Could you check a few things on this model? Use its own coordinates, in mm. A direction names the side the tool comes from. Round coordinates to 2 decimals unless told otherwise and drop trailing zeros. Write each loop counter-clockwise with the first axis right and the second up, starting at its lowest first coordinate (ties: lowest second). Pieces come first, ordered by that corner, then holes.
```python
from build123d import *

# Parameters (mm, degrees)
EXTRUDE_1_DEPTH     = 25
SKETCH_2_R          = 1.75
CUT_EXTRUDE_1_DEPTH = 34
SHELL_1_T           = -2
FILLET_1_R          = 10
FILLET_2_R          = 3
FILLET_3_R          = 5
SKETCH_4_W          = 82
SKETCH_4_H          = 126.745531776
CUT_EXTRUDE_2_DEPTH = 23
FILLET_4_R          = 2
SKETCH_5_W          = 173.89587329
SKETCH_5_H          = 52
CUT_EXTRUDE_3_DEPTH = 23
FILLET_5_R          = 2
SKETCH_6_R          = 4
EXTRUDE_2_DEPTH     = 4
SKETCH_7_R          = 2.5
CUT_EXTRUDE_4_DEPTH = 6
FILLET_6_R          = 5


with BuildPart() as part:
    # Эскиз1 → Бобышка-Вытянуть1 (new body)
    with BuildSketch(Plane.XY):
        Polygon((-52.5, 30), (-45, 37.5), (45, 37.5), (52.5, 30), (52.5, -30), (45, -37.5), (-45, -37.5), (-52.5, -30), align=None)
    extrude(amount=EXTRUDE_1_DEPTH)

    # Эскиз2 → Вырез-Вытянуть1 (cut)
    with BuildSketch(Plane.XY.offset(25)):
        with Locations((-45.214466094, 30.214466094)):
            Circle(SKETCH_2_R)
        with Locations(Location((45.214466094, 30.214466094, 0), (0, 0, 180))):
            Circle(SKETCH_2_R)
        with Locations((45.214466094, -30.214466094)):
            Circle(SKETCH_2_R)
        with Locations(Location((-45.214466094, -30.214466094, 0), (0, 0, 180))):
            Circle(SKETCH_2_R)
    extrude(amount=-CUT_EXTRUDE_1_DEPTH, mode=Mode.SUBTRACT)

    # Оболочка1
    shell_1_openings = [part.faces().sort_by_distance(p)[0] for p in [
        (0, 0, 25),
    ]]
    offset(amount=SHELL_1_T, openings=shell_1_openings, kind=Kind.INTERSECTION)

    # Скругление1
    # the kernel refuses this fillet: 10 mm, written as the material it adds along each edge
    with BuildSketch(Plane(origin=(-45.74479618, -33.926776695, 2), x_dir=(0.7071067811865442, -0.7071067811865507, 0), z_dir=(0, 0, 1)), Plane(origin=(48.926776695, -30.74479618, 2), x_dir=(0.7071067811865482, 0.7071067811865467, 0), z_dir=(0, 0, 1)), Plane(origin=(45.74479618, 33.926776695, 2), x_dir=(-0.707106781186546, 0.7071067811865492, 0), z_dir=(0, 0, 1)), Plane(origin=(-48.926776695, 30.74479618, 2), x_dir=(-0.7071067811865508, -0.7071067811865444, 0), z_dir=(0, 0, 1))) as fillet_1_piece_1:
        with BuildLine():
            CenterArc((11.477032042, 3.794412555), FILLET_1_R, 183.312134334, 18.986942704)
            Line((1.493736012, 3.21665797), (1.294070091, 3.205102878))
            ThreePointArc((1.294070091, 3.205102878), (0.969771845, 1.504817982), (-0.12, 0.16))
            Line((-0.12, 0.16), (0, -0.2))
            ThreePointArc((0, -0.2), (1.112436867, -0.2), (2.039830568, -0.075888251))
            Line((2.039830568, -0.075888251), (2.224873734, 0))
        make_face()
    extrude(amount=23)
    with BuildSketch(Plane(origin=(-48.926776695, -30.74479618, 2), x_dir=(0.34351243985929386, 0.9391481265816991, 0), z_dir=(0, 0, 1)), Plane(origin=(45.74479618, -33.926776695, 2), x_dir=(-0.9391481265817004, 0.34351243985929, 0), z_dir=(0, 0, 1)), Plane(origin=(48.926776695, 30.74479618, 2), x_dir=(-0.3435124398592874, -0.9391481265817014, 0), z_dir=(0, 0, 1)), Plane(origin=(-45.74479618, 33.926776695, 2), x_dir=(0.9391481265817011, -0.34351243985928803, 0), z_dir=(0, 0, 1))) as fillet_1_piece_2:
        with BuildLine():
            CenterArc((8.275322434, 8.811292173), FILLET_1_R, 222.791938952, 18.986942704)
            Line((0.937067943, 2.017911495), (0.790302854, 1.882043882))
            ThreePointArc((0.790302854, 1.882043882), (0.287138375, 1.093191354), (-0.181395597, 0.084235607))
            Line((-0.181395597, 0.084235607), (0.094575114, -0.176225843))
            ThreePointArc((0.094575114, -0.176225843), (1.773283379, 0.245765435), (3.451991644, -0.176225843))
            Line((3.451991644, -0.176225843), (3.546566758, 0))
        make_face()
    extrude(amount=23)

    # Скругление2
    fillet_2_edges = [part.edges().sort_by_distance(p)[0] for p in [
        (-50.5, 29.171572875, 13.5),
        (-44.171572875, 35.5, 13.5),
        (-44.171572875, -35.5, 13.5),
        (-50.5, -29.171572875, 13.5),
        (44.171572875, -35.5, 13.5),
        (50.5, -29.171572875, 13.5),
        (50.5, 29.171572875, 13.5),
        (44.171572875, 35.5, 13.5),
    ]]
    fillet(fillet_2_edges, radius=FILLET_2_R)

    # Скругление3
    fillet_3_edges = [part.edges().sort_by_distance(p)[0] for p in [
        (45, 37.5, 12.5),
        (52.5, 30, 12.5),
        (52.5, -30, 12.5),
        (45, -37.5, 12.5),
        (-45, -37.5, 12.5),
        (-52.5, -30, 12.5),
        (-52.5, 30, 12.5),
        (-45, 37.5, 12.5),
    ]]
    fillet(fillet_3_edges, radius=FILLET_3_R)

    # Эскиз4 → Вырез-Вытянуть2 (cut)
    with BuildSketch(Plane.XY.offset(25)):
        Rectangle(SKETCH_4_W, SKETCH_4_H)
    extrude(amount=-CUT_EXTRUDE_2_DEPTH, mode=Mode.SUBTRACT)

    # Скругление4
    # the kernel refuses this fillet: 2 mm, written as the material it takes off along each edge
    with BuildSketch(Plane(origin=(41, -34.605706623, 2), x_dir=(0, -1, 0), z_dir=(0, 0, 1)), Plane(origin=(41, 34.605706623, 26.756559814), x_dir=(0, 1, 0), z_dir=(0, 0, -1))) as fillet_4_piece_1:
        with BuildLine():
            CenterArc((0.702623926, 2), FILLET_4_R, 235.828901177, 34.171098823)
            ThreePointArc((-0.420708294, 0.345272009), (-0.20250821, 0.18219615), (0, 0))
            Line((0, 0), (0.702623926, 0))
        make_face()
    extrude(amount=24.756559814, mode=Mode.SUBTRACT)
    with BuildSketch(Plane(origin=(41, -37.5, 30.118447555), x_dir=(0.9999997651545144, 0.0006853400003404547, 0), z_dir=(0, 0, -1)), Plane(origin=(-41, -37.5, 2), x_dir=(-0.9999997651545144, 0.0006853400003439418, 0), z_dir=(0, 0, 1)), Plane(origin=(41, 37.5, 2), x_dir=(0.9999997651545144, -0.0006853400003439394, 0), z_dir=(0, 0, 1))) as fillet_4_piece_2:
        with BuildLine():
            CenterArc((2.001370787, -1.999470741), FILLET_4_R, 88.681844886, 91.357422207)
            Line((0.001371257, -2.000841421), (-0.198628696, -2.000978489))
            Line((-0.198628696, -2.000978489), (-0.199999953, -0.000137068))
            Line((-0.199999953, -0.000137068), (-0.000137068, 0.199999953))
            ThreePointArc((-0.000137068, 0.199999953), (1.928794667, 0.201321927), (2.051979846, 0.199947074))
            Line((2.051979846, 0.199947074), (2.047379022, 0))
        make_face()
    extrude(amount=28.118447555, mode=Mode.SUBTRACT)
    with BuildSketch(Plane(origin=(-41, -34.605706623, 2), x_dir=(0, -1, 0), z_dir=(0, 0, 1))) as fillet_4_piece_3:
        with BuildLine():
            CenterArc((0.702623926, -2), FILLET_4_R, 90, 34.171098823)
            ThreePointArc((-0.420708294, -0.345272009), (-0.20250821, -0.18219615), (0, 0))
            Line((0, 0), (0.702623926, 0))
        make_face()
    extrude(amount=24.756559814, mode=Mode.SUBTRACT)
    with BuildSketch(Plane(origin=(-41, 34.605706623, 26.756559814), x_dir=(-0.6343994710235763, -0.7730053758965758, 0), z_dir=(0, 0, -1))) as fillet_4_piece_4:
        with BuildLine():
            CenterArc((0.72566687, 1.991754999), FILLET_4_R, 230.624541426, 34.171098823)
            Line((-0.543132072, 0.445744247), (0, 0))
            ThreePointArc((0, 0), (0.272125076, 0.012367502), (0.544250153, 0))
        make_face()
    extrude(amount=24.756559814, mode=Mode.SUBTRACT)
    with BuildSketch(Plane(origin=(-41, 37.5, 30.118447555), x_dir=(0, -1, 0), z_dir=(0, 0, -1))) as fillet_4_piece_5:
        with BuildLine():
            CenterArc((2.00084189, 2), FILLET_4_R, 178.642577793, 91.357422207)
            Line((0.001403151, 2.047378541), (-0.198540723, 2.052116395))
            ThreePointArc((-0.198540723, 2.052116395), (-0.2, 1.928932188), (-0.2, 0))
            Line((-0.2, 0), (0, -0.2))
            Line((0, -0.2), (2.00084189, -0.2))
            Line((2.00084189, -0.2), (2.00084189, 0))
        make_face()
    extrude(amount=28.118447555, mode=Mode.SUBTRACT)

    # Эскиз5 → Вырез-Вытянуть3 (cut)
    with BuildSketch(Plane.XY.offset(25)):
        Rectangle(SKETCH_5_W, SKETCH_5_H)
    extrude(amount=-CUT_EXTRUDE_3_DEPTH, mode=Mode.SUBTRACT)

    # Скругление5
    # the kernel refuses this fillet: 2 mm, written as the material it takes off along each edge
    with BuildSketch(Plane(origin=(49.605706623, -26, 26.756559814), x_dir=(1, 0, 0), z_dir=(0, 0, -1)), Plane(origin=(-49.605706623, -26, 2), x_dir=(-1, 0, 0), z_dir=(0, 0, 1))) as fillet_5_piece_1:
        with BuildLine():
            CenterArc((0.702623926, 2), FILLET_5_R, 235.828901177, 34.171098823)
            ThreePointArc((-0.420708294, 0.345272009), (-0.20250821, 0.18219615), (0, 0))
            Line((0, 0), (0.702623926, 0))
        make_face()
    extrude(amount=24.756559814, mode=Mode.SUBTRACT)
    with BuildSketch(Plane(origin=(52.5, -26, 2), x_dir=(-0.0006853400003439216, -0.9999997651545144, 0), z_dir=(0, 0, 1)), Plane(origin=(52.5, 26, 30.118447555), x_dir=(-0.0006853400003439287, 0.9999997651545144, 0), z_dir=(0, 0, -1)), Plane(origin=(-52.5, -26, 30.118447555), x_dir=(0.0006853400003404618, -0.9999997651545144, 0), z_dir=(0, 0, -1)), Plane(origin=(-52.5, 26, 2), x_dir=(0.0006853400003404558, 0.9999997651545144, 0), z_dir=(0, 0, 1))) as fillet_5_piece_2:
        with BuildLine():
            CenterArc((2.001370787, -1.999470741), FILLET_5_R, 88.681844886, 91.357422207)
            Line((0.001371257, -2.000841421), (-0.198628696, -2.000978489))
            Line((-0.198628696, -2.000978489), (-0.199999953, -0.000137068))
            Line((-0.199999953, -0.000137068), (-0.000137068, 0.199999953))
            ThreePointArc((-0.000137068, 0.199999953), (1.928794667, 0.201321927), (2.051979846, 0.199947074))
            Line((2.051979846, 0.199947074), (2.047379022, 0))
        make_face()
    extrude(amount=28.118447555, mode=Mode.SUBTRACT)
    with BuildSketch(Plane(origin=(49.605706623, 26, 26.756559814), x_dir=(-0.7730053758965695, 0.6343994710235842, 0), z_dir=(0, 0, -1))) as fillet_5_piece_3:
        with BuildLine():
            CenterArc((0.72566687, 1.991754999), FILLET_5_R, 230.624541426, 34.171098823)
            Line((-0.543132072, 0.445744247), (0, 0))
            ThreePointArc((0, 0), (0.272125076, 0.012367502), (0.544250153, 0))
        make_face()
    extrude(amount=24.756559814, mode=Mode.SUBTRACT)
    with BuildSketch(Plane(origin=(-49.605706623, 26, 2), x_dir=(-1, 0, 0), z_dir=(0, 0, 1))) as fillet_5_piece_4:
        with BuildLine():
            CenterArc((0.702623926, -2), FILLET_5_R, 90, 34.171098823)
            ThreePointArc((-0.420708294, -0.345272009), (-0.20250821, -0.18219615), (0, 0))
            Line((0, 0), (0.702623926, 0))
        make_face()
    extrude(amount=24.756559814, mode=Mode.SUBTRACT)

    # Эскиз6 → Бобышка-Вытянуть2 (add)
    with BuildSketch(Plane.XY.offset(2)):
        with Locations(Location((-38.5, 24.5, 0), (0, 0, 180))):
            Circle(SKETCH_6_R)
        with Locations(Location((19.5, 24.5, 0), (0, 0, 180))):
            Circle(SKETCH_6_R)
        with Locations(Location((19.5, -24.5, 0), (0, 0, 180))):
            Circle(SKETCH_6_R)
        with Locations(Location((-38.5, -24.5, 0), (0, 0, 180))):
            Circle(SKETCH_6_R)
    extrude(amount=EXTRUDE_2_DEPTH)

    # Эскиз7 → Вырез-Вытянуть4 (cut)
    with BuildSketch(Plane.XY.offset(6)):
        with Locations((-38.5, 24.5)):
            Circle(SKETCH_7_R)
        with Locations((19.5, 24.5)):
            Circle(SKETCH_7_R)
        with Locations((19.5, -24.5)):
            Circle(SKETCH_7_R)
        with Locations((-38.5, -24.5)):
            Circle(SKETCH_7_R)
    extrude(amount=-CUT_EXTRUDE_4_DEPTH, mode=Mode.SUBTRACT)

    # Скругление6
    # the kernel refuses this fillet: 5 mm, written as the material it adds along each edge
    with BuildSketch(Plane(origin=(-38.5, 24.5, 2), x_dir=(-1, 0, 0), z_dir=(0, 1, 0))) as fillet_6_piece_1_section:
        with BuildLine():
            CenterArc((8.898979486, 5), FILLET_6_R, 191.536959033, 78.463040967)
            Line((4, 4), (4, 0))
            Line((4, 0), (8.898979486, 0))
        make_face()
    fillet_6_piece_1 = revolve(axis=Axis((-38.5, 24.5, 2), (0, 0, 1)), mode=Mode.PRIVATE)
    fillet_6_piece_1 = fillet_6_piece_1 - Plane(origin=(-45.214466094, 30.214466094, 3.119270687), x_dir=(1, 0, 0), z_dir=(0, 0, 1)) * Cylinder(1.75, 36, mode=Mode.PRIVATE)
    add(fillet_6_piece_1)
    with BuildSketch(Plane(origin=(-38.5, -24.5, 2), x_dir=(-1, 0, 0), z_dir=(0, 1, 0))) as fillet_6_piece_2_section:
        with BuildLine():
            CenterArc((8.898979486, 5), FILLET_6_R, 191.536959033, 78.463040967)
            Line((4, 4), (4, 0))
            Line((4, 0), (8.898979486, 0))
        make_face()
    fillet_6_piece_2 = revolve(axis=Axis((-38.5, -24.5, 2), (0, 0, 1)), mode=Mode.PRIVATE)
    fillet_6_piece_2 = fillet_6_piece_2 - Plane(origin=(-45.214466094, -30.214466094, 3.119270687), x_dir=(-1, 0, 0), z_dir=(0, 0, 1)) * Cylinder(1.75, 36, mode=Mode.PRIVATE)
    add(fillet_6_piece_2)
    with BuildSketch(Plane(origin=(19.5, -24.5, 2), x_dir=(-1, 0, 0), z_dir=(0, 1, 0))) as fillet_6_piece_3:
        with BuildLine():
            CenterArc((8.898979486, 5), FILLET_6_R, 191.536959033, 78.463040967)
            Line((4, 4), (4, 0))
            Line((4, 0), (8.898979486, 0))
        make_face()
    revolve(axis=Axis((19.5, -24.5, 2), (0, 0, 1)))
    with BuildSketch(Plane(origin=(19.5, 24.5, 2), x_dir=(-1, 0, 0), z_dir=(0, 1, 0))) as fillet_6_piece_4:
        with BuildLine():
            CenterArc((8.898979486, 5), FILLET_6_R, 191.536959033, 78.463040967)
            Line((4, 4), (4, 0))
            Line((4, 0), (8.898979486, 0))
        make_face()
    revolve(axis=Axis((19.5, 24.5, 2), (0, 0, 1)))


solid = part.part
```
Q1. We'd pull the mould along X, two halves only. Please class faces 1 (the cylindrical face through (-42.605, 27.521, 13.68)), 2 (the cylindrical face through (41.619, 36.946, 13.339)), 3 (the cylindrical face through (-52.11, -29.87, 12.68)), 4 (the cylindrical face through (52.11, 29.87, 12.68)): pulls with the +X half, pulls with the -X half, needs draft (parallel to the pull), parting line crosses it, or undercut.
Q2. If I drill on L1, parallel to Z at x = 21.5, y = 22; L2, parallel to Y at x = 19.5, z = 3.3; L3, parallel to X at y = 29, z = 18.25, over which ranges is the centre line in solid material (lowest first)?
Q3. Imagine slicing it at C-C, the plane z = 16.25. Count the separate pieces of the cut face and the enclosed holes in it, then the cut area to 3 significant figures.
Q4. Imagine slicing it at A-A, the plane y = -24.5. Write out the boundary of the cut face in (x, z).
Q5. On a 3-axis mill with a long thin cutter (end or side, diameter ignored), from which of +Z, -Z, +X, -X, +Y, -Y can I reach the whole of each face in a straight line? I mean faces 5 (the cylindrical face through (44.82, 37.13, 12.68)), 6 (the flat face through (-1, 1, 2)), 7 (the cylindrical face through (-41.619, -36.946, 13.339)). Say none if no direction works.
Q6. Imagine slicing it at B-B, the plane x = 19.5. Write out the boundary of the cut face in (y, z), then the cut area to 3 significant figures.
Q7. I'm going to push flat-ended pins straight in: pin 1 Ø9 at (x, y) = (20.5, -24) entering from +Z; pin 2 Ø3 at (x, y) = (18, 10.5) entering from +Z. Where does each tip first touch, or does it pass through?
Q8. Imagine slicing it at D-D, the plane y = 11. Write out the boundary of the cut face in (x, z), then the cut area to 3 significant figures.
Results found:
1. face 1: undercut
1. face 2: undercut
1. face 3: pulls with the -X half
1. face 4: pulls with the +X half
2. L1: z = 0 to 6
2. L2: y = -30.04 to -27, -22 to -18.96, 18.96 to 22, 27 to 30.04
2. L3: x = -52.38 to -46.47, -43.95 to -41.67, 41.67 to 43.95, 46.47 to 52.38
3. separate pieces: 4
3. enclosed holes: 4
3. area: 318 mm2
4. outline: (-52.5, 0) - (-41, 0) - (-41, 6) - (-42.5, 6) arc R5 cw to (-47.4, 2) - (-52.5, 2) - close; (-36, 0) - (17, 0) - (17, 6) - (15.5, 6) arc R5 cw to (10.6, 2) - (-29.6, 2) arc R5 cw to (-34.5, 6) - (-36, 6) - close; (22, 0) - (52.5, 0) - (52.5, 2) - (28.4, 2) arc R5 cw to (23.5, 6) - (22, 6) - close
5. face 5: +Z, -Z, +X, +Y
5. face 6: +Z
5. face 7: +Z, -Y
6. outline: (-37.5, 0) - (-27, 0) - (-27, 6) - (-28.5, 6) arc R5 cw to (-33.4, 2) - (-37.5, 2) - close; (-22, 0) - (22, 0) - (22, 6) - (20.5, 6) arc R5 cw to (15.6, 2) - (-15.6, 2) arc R5 cw to (-20.5, 6) - (-22, 6) - close; (27, 0) - (37.5, 0) - (37.5, 2) - (33.4, 2) arc R5 cw to (28.5, 6) - (27, 6) - close
6. area: 174 mm2
7. pin 1: stops at z = 6
7. pin 2: stops at z = 2
8. outline: (-52.5, 0) - (52.5, 0) - (52.5, 2) - (-52.5, 2) - close
8. area: 210 mm2
